Part model, mm, in its own coordinate system. Face numbers are marked on the shaded views. A direction names the side the tool comes from. Give positions to 0.01 mm unless a question says otherwise; leave off trailing zeros. Order: outer loops, then holes, each group sorted by start corner. A loop starts at its lowest first (then second) coordinate and runs counter-clockwise, first axis right, second up. Notation, with made-up numbers: (27.25, -27) - (79.25, -27) arc R25 ccw to (79.25, 2) - close; hole circle Ø1 at (-11.75, 33). An arc over 180 degrees is marked (long way). One line per item, written item: value.
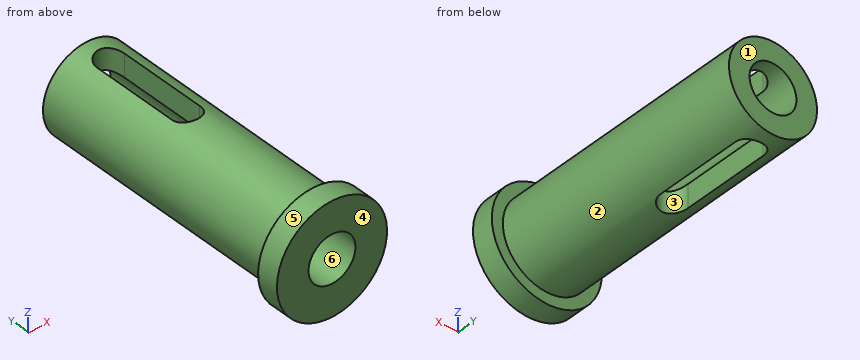
```python
from build123d import *

# Parameters (mm, degrees)
SKETCH1_R                 = 3.175
BOSS_EXTRUDE1_DEPTH       = 1.27
SKETCH2_R                 = 2.54
BOSS_EXTRUDE2_DEPTH       = 15.24
TAP_DRILL_FOR_6_32_TAP1_D = 2.7051
CUT_EXTRUDE1_DEPTH        = 18.109685853
CUT_EXTRUDE1_DEPTH_BACK   = 18.109685853


with BuildPart() as part:
    # Sketch1 → Boss-Extrude1 (new body)
    with BuildSketch(Plane(origin=(0, 0, 0), x_dir=(1, 0, 0), z_dir=(0, 1, 0))):
        with Locations(Location((0, 0, 0), (0, 0, 270))):
            Circle(SKETCH1_R)
    extrude(amount=BOSS_EXTRUDE1_DEPTH)

    # Sketch2 → Boss-Extrude2 (add)
    with BuildSketch(Plane(origin=(0, 1.27, 0), x_dir=(1, 0, 0), z_dir=(0, 1, 0))):
        with Locations(Location((0, 0, 0), (0, 0, 90))):
            Circle(SKETCH2_R)
    extrude(amount=BOSS_EXTRUDE2_DEPTH)

    # Tap Drill for #6-32 Tap1 (through all)
    with Locations(Plane(origin=(0, 16.51, 0), x_dir=(1, 0, 0), z_dir=(0, 1, 0))):
        with Locations((0, 0)):
            Hole(TAP_DRILL_FOR_6_32_TAP1_D / 2)

    # Sketch6 → Cut-Extrude1 (cut, two sides: drawn at the far end of the back side and taken through both)
    with BuildSketch(Plane.XY.offset(-CUT_EXTRUDE1_DEPTH_BACK)):
        with BuildLine():
            Line((0.79375, 14.9225), (0.79375, 9.8425))
            ThreePointArc((0.79375, 9.8425), (0, 9.04875), (-0.79375, 9.8425))
            Line((-0.79375, 9.8425), (-0.79375, 14.9225))
            ThreePointArc((-0.79375, 14.9225), (0, 15.71625), (0.79375, 14.9225))
        make_face()
    extrude(amount=CUT_EXTRUDE1_DEPTH + CUT_EXTRUDE1_DEPTH_BACK, mode=Mode.SUBTRACT)


solid = part.part
```
1) Cut at A-A, the plane y = 10. Give the cut face in (x, z).
Outcome:
outline: (-0.79, -2.41) - (-0.79, -1.1) arc R1.35 cw to (-0.79, 1.1) - (-0.79, 2.41) arc R2.54 ccw to start; (0.79, -2.41) arc R2.54 ccw to (0.79, 2.41) - (0.79, 1.1) arc R1.35 cw to (0.79, -1.1) - close
2) Pin check, flat tips, straight feed: pin 1 (2 mm diameter, centred on y = 4.5, z = -0.5, fed in from -X); pin 2 (1.1 mm diameter, centred on y = 13.5, z = -1.5, fed in from +X); pin 3 (0.7 mm diameter, centred on y = 12.5, z = 2, fed in from -X). Stop position of each tip, or through.
Outcome:
pin 1: stops at x = -2.54
pin 2: stops at x = 2.36
pin 3: stops at x = -1.93
3) Which spindle directions (+Z, -Z, +X, -X, +Y, -Y) get a long thin tool onto all of the face, cutting with end or side? Do the marked faces 1, 2 and 3. Say none if no direction does.
Outcome:
face 1: +Z, -Z, +X, -X, +Y
face 2: +Y
face 3: +Z, -Z
4) Mould opens along X. For the marked faces 4, 5 and 6 say: released by +X, released by -X, zero draft, split by the parting line, or undercut.
Outcome:
face 4: zero draft
face 5: split by the parting line
face 6: undercut
5) Drill centre lines: line 1 along X through (y, z) = (11.5, -0.25); line 2 along Y through (x, z) = (0.5, -1.75). Where is each one in solid material? Low to high. Write a range as from..to.
Outcome:
line 1: x = -2.53..-1.33, 1.33..2.53
line 2: y = 0..9.23, 15.54..16.51
6) Cut at D-D, the plane y = 1.5. Give the cut face in (x, z), then the cut area to 3 significant figures.
Outcome:
outline: circle Ø5.08 at (0, 0); hole circle Ø2.71 at (0, 0)
area: 14.5 mm^2
7) Cut at B-B, the plane z = 0. Give the cut face in (x, y) (3 decimals).
Outcome:
outline: (-3.175, 0) - (-1.353, 0) - (-1.353, 16.51) - (-2.54, 16.51) - (-2.54, 1.27) - (-3.175, 1.27) - close; (1.353, 0) - (3.175, 0) - (3.175, 1.27) - (2.54, 1.27) - (2.54, 16.51) - (1.353, 16.51) - close
8) Cut at C-C, the plane x = 0. Give the cut face in (y, z) (3 decimals).
Outcome:
outline: (0, -3.175) - (1.27, -3.175) - (1.27, -2.54) - (9.049, -2.54) - (9.049, -1.353) - (0, -1.353) - close; (0, 1.353) - (9.049, 1.353) - (9.049, 2.54) - (1.27, 2.54) - (1.27, 3.175) - (0, 3.175) - close; (15.716, -2.54) - (16.51, -2.54) - (16.51, -1.353) - (15.716, -1.353) - close; (15.716, 1.353) - (16.51, 1.353) - (16.51, 2.54) - (15.716, 2.54) - close
